Check sheet for the drawn part. Datum: minimum x, y, z corner. Units: mm. Round coordinates to 2 decimals unless told otherwise and drop trailing zeros. Write each loop counter-clockwise with the first axis right and the second up, starting at its lowest first coordinate (ties: lowest second). Pieces come first, ordered by that corner, then holes. Notation, with made-up numbers: (34.5, 8) -> (44.5, 8) arc R32 ccw to (44.5, 34) -> close; hole circle Ø5 at (-1, -7). An arc over 180 degrees is marked (long way). Use a Markdown table: item, result.
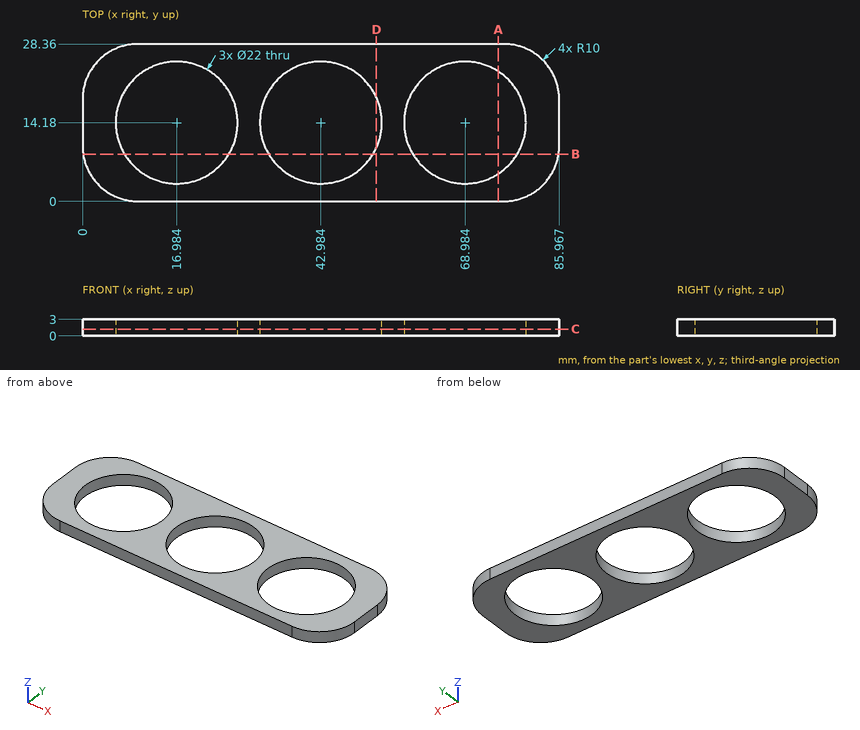
(1) Section check C-C on z = 1.2. Record the cut outline in (x, y).
A:
| item | result |
|---|---|
| outline | (0, 10) arc R10 ccw to (10, 0) -> (75.97, 0) arc R10 ccw to (85.97, 10) -> (85.97, 18.36) arc R10 ccw to (75.97, 28.36) -> (10, 28.36) arc R10 ccw to (0, 18.36) -> close; hole circle Ø22 at (16.98, 14.18); hole circle Ø22 at (42.98, 14.18); hole circle Ø22 at (68.98, 14.18) |
(2) Section check A-A on x = 75. Record the cut outline in (y, z).
A:
| item | result |
|---|---|
| outline | (0, 0) -> (4.97, 0) -> (4.97, 3) -> (0, 3) -> close; (23.39, 0) -> (28.36, 0) -> (28.36, 3) -> (23.39, 3) -> close |
(3) Section check B-B on y = 8.5. Record the cut outline in (x, z).
A:
| item | result |
|---|---|
| outline | (0.11, 0) -> (7.56, 0) -> (7.56, 3) -> (0.11, 3) -> close; (26.4, 0) -> (33.56, 0) -> (33.56, 3) -> (26.4, 3) -> close; (52.4, 0) -> (59.56, 0) -> (59.56, 3) -> (52.4, 3) -> close; (78.4, 0) -> (85.85, 0) -> (85.85, 3) -> (78.4, 3) -> close |
(4) Thickness scan on line 1 (X direction, y = 21.5, z = 1.05) (1 decimal); line 2 (X direction, y = 18.5, z = 2.6) (1 decimal); line 3 (Y direction, x = 72.5, z = 1.4). Record the ranges inside material, lowest first.
A:
| item | result |
|---|---|
| line 1 | x = 0.5 to 8.8, 25.2 to 34.8, 51.2 to 60.8, 77.2 to 85.5 |
| line 2 | x = 0 to 6.9, 27.1 to 32.9, 53.1 to 58.9, 79.1 to 86 |
| line 3 | y = 0 to 3.76, 24.6 to 28.36 |
(5) Section check D-D on x = 53. Record the cut outline in (y, z).
A:
| item | result |
|---|---|
| outline | (0, 0) -> (9.63, 0) -> (9.63, 3) -> (0, 3) -> close; (18.73, 0) -> (28.36, 0) -> (28.36, 3) -> (18.73, 3) -> close |
